Geometry: final body of the model. Coordinates: model frame, mm. A direction names the side the tool comes from. Give positions to 0.01 mm unless a question says otherwise; leave off trailing zeros. Order: outer loops, then holes, each group sorted by start corner. A loop starts at its lowest first (then second) coordinate and runs counter-clockwise, first axis right, second up. Notation, with made-up numbers: (17, 18.25) - (75, 18.25) arc R17 ccw to (75, 36.25) - close; hole circle Ø4 at (12.25, -23.5). An arc over 180 degrees is marked (long way). Write item = value, one per line. Start each with the question number.
from build123d import *

# Parameters (mm, degrees)
SKETCH_1_R          = 20
EXTRUDE_1_DEPTH     = 10
SKETCH_2_R          = 3
CUT_EXTRUDE_1_DEPTH = 10
SKETCH_3_R          = 4
CUT_EXTRUDE_2_DEPTH = 4
FILLET_1_R          = 0.5
CHAMFER_1_SIZE      = 0.5
CHAMFER_2_SIZE      = 0.5
SKETCH_6_R          = 1.5
CUT_EXTRUDE_7_DEPTH = 6


with BuildPart() as part:
    # 草图1 → 凸台-拉伸1 (new body)
    with BuildSketch(Plane.XY):
        Circle(SKETCH_1_R)
    extrude(amount=EXTRUDE_1_DEPTH)

    # 草图2 → 切除-拉伸1 (cut)
    with BuildSketch(Plane.XY.offset(10)):
        Circle(SKETCH_2_R)
    extrude(amount=-CUT_EXTRUDE_1_DEPTH, mode=Mode.SUBTRACT)

    # 草图3 → 切除-拉伸2 (cut)
    with BuildSketch(Plane.XY.offset(10)):
        Circle(SKETCH_3_R)
    extrude(amount=-CUT_EXTRUDE_2_DEPTH, mode=Mode.SUBTRACT)

    # 圆角1
    fillet_1_edges = [part.edges().sort_by_distance(p)[0] for p in [
        (-20, 0, 0),
        (-20, 0, 10),
    ]]
    fillet(fillet_1_edges, radius=FILLET_1_R)

    # 倒角1
    chamfer_1_edges = [part.edges().sort_by_distance(p)[0] for p in [
        (-3, 0, 0),
    ]]
    chamfer(chamfer_1_edges, length=CHAMFER_1_SIZE)

    # 倒角2
    chamfer_2_edges = [part.edges().sort_by_distance(p)[0] for p in [
        (-4, 0, 10),
    ]]
    chamfer(chamfer_2_edges, length=CHAMFER_2_SIZE)

    # 草图6 → 切除-拉伸7 (cut)
    with BuildSketch(Plane.XY.offset(10)):
        with Locations((-8, 4.353810299)):
            Circle(SKETCH_6_R)
        with Locations((8, -5.646189701)):
            Circle(SKETCH_6_R)
    extrude(amount=-CUT_EXTRUDE_7_DEPTH, mode=Mode.SUBTRACT)


solid = part.part
Q1. Contact query for flat-ended pins moving along their axis: pin 1 (1.5 mm diameter, centred on x = 2, z = 5, fed in from -Y); pin 2 (2 mm diameter, centred on x = -7, z = 5.5, fed in from +Y); pin 3 (5 mm diameter, centred on y = 3.5, z = 4, fed in from +X) (3 decimals). Output: stop coordinate, or through.
Q2. Set-up query: faces 4 (the cylindrical face through (-3, 0, 3)), 5 (the cylindrical face through (-0.867, -3.905, 7.774)). Return all of +Z, -Z, +X, -X, +Y, -Y with unobstructed straight access to the full face (end or side cutting, diameter ignored); none if empty.
Q3. Section B-B, the plane z = 6.5. Return the cut outline in (x, y).
Q4. Pull-direction query (Y, two-part tool) for faces 1 (the cylindrical face through (-4.336, -19.524, 4.937)), 2 (the flat face through (0, -4, 0)), 3 (the flat face through (1, 3, 6)); classes: +Y half, -Y half, draft (parallel to the pull), parting line (faces both ways), or undercut.
Q5. Section A-A, the plane y = 0. Return the cut outline in (x, z).
Q6. Material intervals for line 1 along Y through (x, z) = (0, 8.35); line 2 along Y through (x, z) = (9, 7.5); line 3 along X through (y, z) = (-1, 0.5), sorted ascending. Write a range as from..to.
The answers:
q1.pin_1 = -19.96
q1.pin_2 = 19.08
q1.pin_3 = 19.975
q2.face_4 = +Z, -Z
q2.face_5 = +Z
q3.outline = circle Ø40 at (0, 0); hole circle Ø3 at (-8, 4.35); hole circle Ø8 at (0, 0); hole circle Ø3 at (8, -5.65)
q4.face_1 = parting line
q4.face_2 = draft
q4.face_3 = undercut
q5.outline = (-20, 0.5) arc R0.5 ccw to (-19.5, 0) - (-3.5, 0) - (-3, 0.5) - (-3, 6) - (-4, 6) - (-4, 9.5) - (-4.5, 10) - (-19.5, 10) arc R0.5 ccw to (-20, 9.5) - close; (3, 0.5) - (3.5, 0) - (19.5, 0) arc R0.5 ccw to (20, 0.5) - (20, 9.5) arc R0.5 ccw to (19.5, 10) - (4.5, 10) - (4, 9.5) - (4, 6) - (3, 6) - close
q6.line_1 = -20..-4, 4..20
q6.line_2 = -17.86..-6.76, -4.53..17.86
q6.line_3 = -19.97..-2.83, 2.83..19.97
